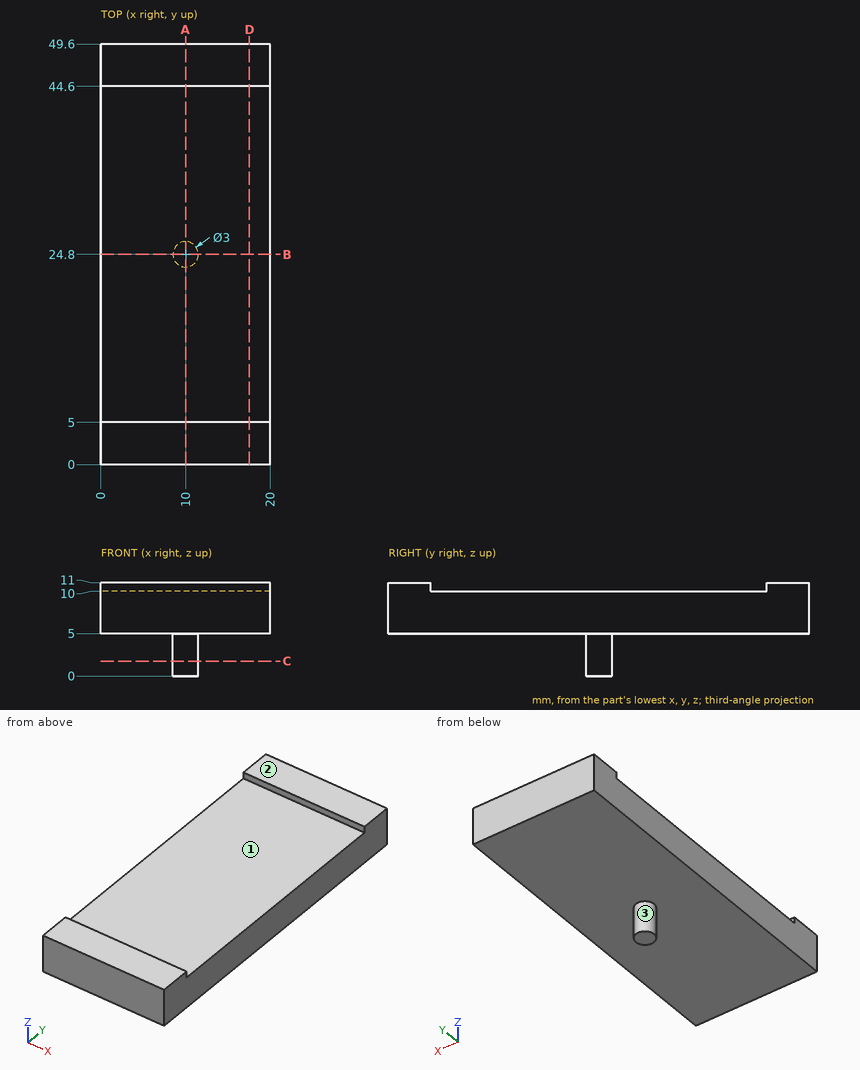
Geometry check sheet. Reference: drawing and pictorial views, mm from the part's lowest x, y, z. Coordinates: 2 decimals unless noted, no trailing zeros. Write each loop counter-clockwise with the first axis right and the second up, starting at its lowest first coordinate (ties: lowest second). Pieces come first, ordered by that corner, then holes. Notation, with made-up numbers: (14.25, 64) - (73.25, 64) arc R16 ccw to (73.25, 79) - close; hole circle Ø6 at (1, 79.25). An arc over 180 degrees is marked (long way). One line per question, with ' | ' between items. Start each with the question number.
1. Gauge pin test, flat end, axial feed: P1, Ø10, axis at x = 11.5, y = 30, coming from the +Z side. Record the tip position at first contact, or that the pin passes through.
2. Section check D-D (x = 17.5). Enter the section's corners in (y, z), plus the area to 3 significant figures.
3. Material ranges on line 1 along Y through (x, z) = (2.25, 10.25); line 2 along Z through (x, y) = (5, 26); line 3 along Z through (x, y) = (1.5, 45), recorded low to high.
4. Draft check along Y on the marked faces 1, 2 and 3. Enter one of: released by +Y, released by -Y, zero draft, split by the parting line, or undercut.
5. Section check C-C (z = 1.75). Enter the section's corners in (x, y), plus the area to 3 significant figures.
6. Section check B-B (y = 24.8). Enter the section's corners in (x, z), plus the area to 3 significant figures.
7. Section check A-A (x = 10). Enter the section's corners in (y, z), plus the area to 3 significant figures.
Computed values:
1) P1: z = 10
2) outline: (0, 5) - (49.6, 5) - (49.6, 11) - (44.6, 11) - (44.6, 10) - (5, 10) - (5, 11) - (0, 11) - close | area: 258 mm²
3) line 1: 0 to 5, 44.6 to 49.6 | line 2: 5 to 10 | line 3: 5 to 11
4) face 1: undercut | face 2: zero draft | face 3: split by the parting line
5) outline: circle Ø3 at (10, 24.8) | area: 7.07 mm²
6) outline: (0, 5) - (8.5, 5) - (8.5, 0) - (11.5, 0) - (11.5, 5) - (20, 5) - (20, 10) - (0, 10) - close | area: 115 mm²
7) outline: (0, 5) - (23.3, 5) - (23.3, 0) - (26.3, 0) - (26.3, 5) - (49.6, 5) - (49.6, 11) - (44.6, 11) - (44.6, 10) - (5, 10) - (5, 11) - (0, 11) - close | area: 273 mm²
